```python
from build123d import *

# Parameters (mm, degrees)
SKETCH_1_W          = 50
SKETCH_1_H          = 50
SKETCH_1_R          = 2
SKETCH_1_R_2        = 1.5
EXTRUDE_1_DEPTH     = 2
SKETCH_3_W          = 33.603167957
SKETCH_3_H          = 55.181672871
CUT_EXTRUDE_2_DEPTH = 10


with BuildPart() as part:
    # 草图1 → 凸台-拉伸1 (new body)
    with BuildSketch(Plane.XY):
        Rectangle(SKETCH_1_W, SKETCH_1_H)
        Circle(SKETCH_1_R, mode=Mode.SUBTRACT)
        with Locations((-20, 20)):
            Circle(SKETCH_1_R_2, mode=Mode.SUBTRACT)
        with Locations(Location((20, 20, 0), (0, 0, 180))):
            Circle(SKETCH_1_R_2, mode=Mode.SUBTRACT)
        with Locations((20, -20)):
            Circle(SKETCH_1_R_2, mode=Mode.SUBTRACT)
        with Locations(Location((-20, -20, 0), (0, 0, 180))):
            Circle(SKETCH_1_R_2, mode=Mode.SUBTRACT)
    extrude(amount=EXTRUDE_1_DEPTH)

    # 草图3 → 切除-拉伸2 (cut)
    with BuildSketch(Plane.XY.offset(2)):
        with Locations((16.801583979, -0.050186901)):
            Rectangle(SKETCH_3_W, SKETCH_3_H)
    extrude(amount=-CUT_EXTRUDE_2_DEPTH, mode=Mode.SUBTRACT)


solid = part.part
```
Could you check a few things on this model? Use its own coordinates, in mm. Round coordinates to 2 decimals unless told otherwise and drop trailing zeros. Write each loop counter-clockwise with the first axis right and the second up, starting at its lowest first coordinate (ties: lowest second). Pieces come first, ordered by that corner, then holes. Notation, with made-up numbers: M -10.5,-27.75 L 24.5,-27.75 A34 cw 24.5,4.25 Z; hole C 54,41 d1. An arc over 180 degrees is marked long. Answer in a Markdown table with one row per item. Add a question column.
Q1. Imagine slicing it at C-C (z = 0.95). Please give me the cut outline in (x, y), then the cut area to 3 significant figures.
Q2. Imagine slicing it at A-A (y = -20). Please give me the cut outline in (x, z), then the cut area to 3 significant figures.
Q3. Imagine slicing it at B-B (x = -20). Please give me the cut outline in (y, z).
Q4. If we mould it in two halves opening along X, with no side actions, what happens to faces 1 (the flat face through (-25, 0, 1)), 2 (the cylindrical face through (-21.11, 21.01, 0.99)), 3 (the flat face through (-13, 0, 2)), 4 (the cylindrical face through (-18.89, -21.01, 0.99))? For each: +X half, -X half, draft (parallel to the pull), parting line (faces both ways), or undercut.
Q5. Imagine slicing it at D-D (y = 21). Please give me the cut outline in (x, z), then the cut area to 3 significant figures.
Q6. If I drill on line 1 (Y direction, x = -20, z = 0.8); line 2 (X direction, y = -20, z = 0.55); line 3 (X direction, y = 19.5, z = 1.55), over which ranges is the centre line in solid material (lowest first)? Write a range as from..to.
Values:
| question | item | result |
|---|---|---|
| 1 | outline | M -25,-25 L 0,-25 L 0,-2 A2 cw 0,2 L 0,25 L -25,25 Z; hole C -20,-20 d3; hole C -20,20 d3 |
| 1 | area | 1,230 mm^2 |
| 2 | outline | M -25,0 L -21.5,0 L -21.5,2 L -25,2 Z; M -18.5,0 L 0,0 L 0,2 L -18.5,2 Z |
| 2 | area | 44.0 mm^2 |
| 3 | outline | M -25,0 L -21.5,0 L -21.5,2 L -25,2 Z; M -18.5,0 L 18.5,0 L 18.5,2 L -18.5,2 Z; M 21.5,0 L 25,0 L 25,2 L 21.5,2 Z |
| 4 | face 1 | -X half |
| 4 | face 2 | undercut |
| 4 | face 3 | draft |
| 4 | face 4 | undercut |
| 5 | outline | M -25,0 L -21.12,0 L -21.12,2 L -25,2 Z; M -18.88,0 L 0,0 L 0,2 L -18.88,2 Z |
| 5 | area | 45.5 mm^2 |
| 6 | line 1 | -25..-21.5, -18.5..18.5, 21.5..25 |
| 6 | line 2 | -25..-21.5, -18.5..0 |
| 6 | line 3 | -25..-21.41, -18.59..0 |
